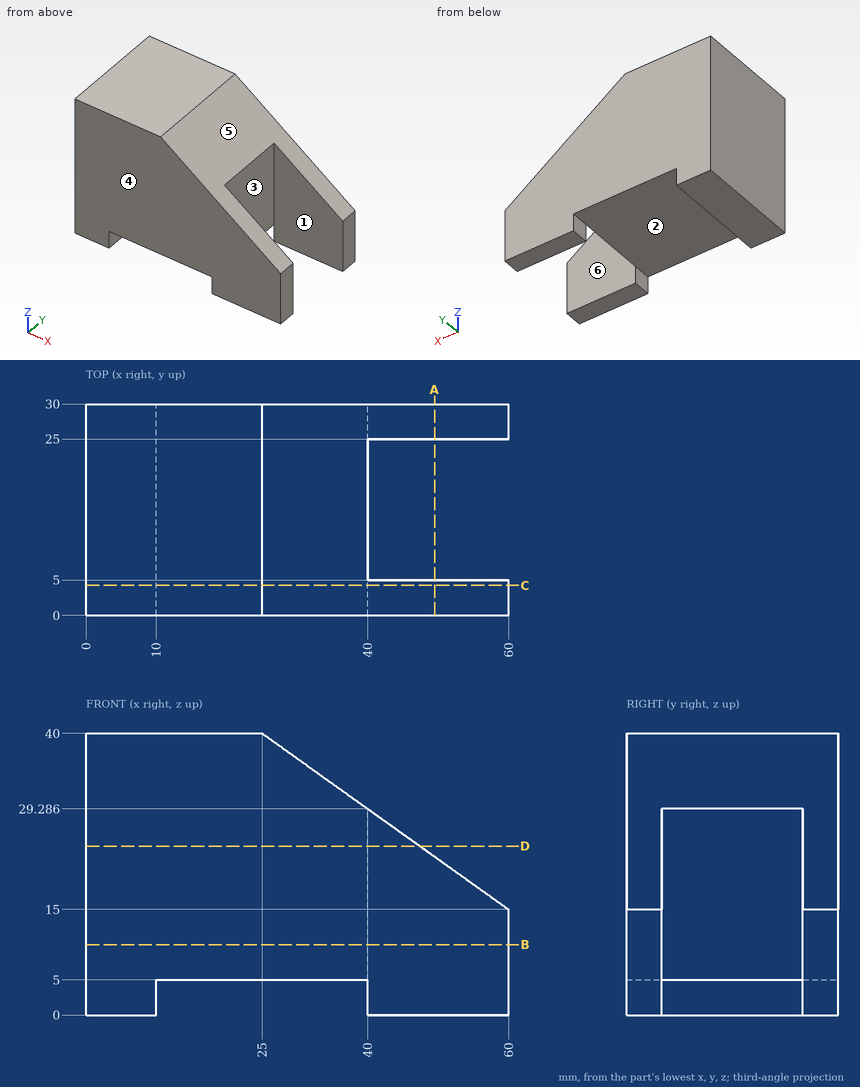
Could you check a few things on this drawing? It's one solid part, dimensions in mm from its lowest x, y, z. A direction names the side the tool comes from. Round coordinates to 2 decimals unless told otherwise and drop trailing zeros. Order: outer loops, then holes, each group sorted by start corner. A loop starts at its lowest first (then second) coordinate and runs counter-clockwise, first axis right, second up. Notation, with made-up numbers: M 42.25,69 L 80.25,69 A11 ccw 80.25,88 Z; hole C 54.5,15.5 d10. An arc over 180 degrees is marked long. Use a Markdown table: item, result.
1) Imagine slicing it at C-C (y = 4.25). List the corners of the cut face in (x, z) for me.
Geometry says:
| item | result |
|---|---|
| outline | M 0,0 L 10,0 L 10,5 L 40,5 L 40,0 L 60,0 L 60,15 L 25,40 L 0,40 Z |
2) On a 3-axis mill with a long thin cutter (end or side, diameter ignored), from which of +Z, -Z, +X, -X, +Y, -Y can I reach the whole of each face in a straight line? I mean the marked faces 5 and 6. Say none if no direction works.
Geometry says:
| item | result |
|---|---|
| face 5 | +Z, +X, +Y, -Y |
| face 6 | +Z, -Z, +X |
3) Imagine slicing it at D-D (z = 24). List the corners of the cut face in (x, y) for me, then the cut area to 3 significant figures.
Geometry says:
| item | result |
|---|---|
| outline | M 0,0 L 47.4,0 L 47.4,5 L 40,5 L 40,25 L 47.4,25 L 47.4,30 L 0,30 Z |
| area | 1,270 mm² |
4) I'm going to push flat-ended pins straight in: P1, Ø6, axis at y = 10.5, z = 21.5, coming from the +X side; P2, Ø1, axis at y = 5, z = 22.5, coming from the +X side; P3, Ø15, axis at x = 29.5, y = 15.5, coming from the -Z side. Where does each tip first touch, or does it pass through?
Geometry says:
| item | result |
|---|---|
| P1 | stops at x = 40 |
| P2 | stops at x = 50.2 |
| P3 | stops at z = 5 |
5) If we mould it in two halves opening along Y, with no side actions, what happens to the marked faces 1, 2, 3 and 4? For each: +Y half, -Y half, draft (parallel to the pull), parting line (faces both ways), or undercut.
Geometry says:
| item | result |
|---|---|
| face 1 | undercut |
| face 2 | draft |
| face 3 | undercut |
| face 4 | -Y half |
6) Imagine slicing it at A-A (x = 49.5). List the corners of the cut face in (y, z) for me, then the cut area to 3 significant figures.
Geometry says:
| item | result |
|---|---|
| outline | M 0,0 L 5,0 L 5,22.5 L 0,22.5 Z; M 25,0 L 30,0 L 30,22.5 L 25,22.5 Z |
| area | 225 mm² |
7) Imagine slicing it at B-B (z = 10). List the corners of the cut face in (x, y) for me.
Geometry says:
| item | result |
|---|---|
| outline | M 0,0 L 60,0 L 60,5 L 40,5 L 40,25 L 60,25 L 60,30 L 0,30 Z |
8) If I drill on line 1 along Z through (x, y) = (16.5, 25); line 2 along X through (y, z) = (14, 23); line 3 along Y through (x, z) = (42, 14), over which ranges is the centre line in solid material (lowest first)?
Geometry says:
| item | result |
|---|---|
| line 1 | z = 5 to 40 |
| line 2 | x = 0 to 40 |
| line 3 | y = 0 to 5, 25 to 30 |
